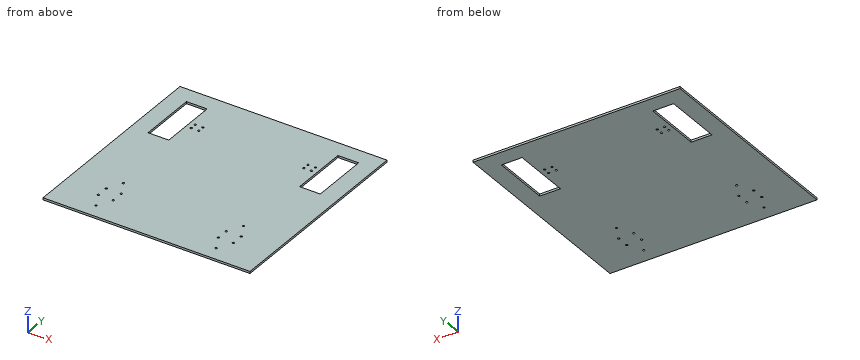
```python
from build123d import *

# Parameters (mm, degrees)
SKETCH1_W           = 500
SKETCH1_H           = 500
SKETCH1_R           = 2.5
SKETCH1_W_2         = 50
SKETCH1_H_2         = 140
BOSS_EXTRUDE1_DEPTH = 5
CUT_EXTRUDE1_START  = -5
SKETCH2_R           = 2.5
CUT_EXTRUDE1_DEPTH  = 5


with BuildPart() as part:
    # Sketch1 → Boss-Extrude1 (new body)
    with BuildSketch(Plane.XY):
        Rectangle(SKETCH1_W, SKETCH1_H)
        with Locations((127, 147.5)):
            Circle(SKETCH1_R, mode=Mode.SUBTRACT)
        with Locations((127, 132.5)):
            Circle(SKETCH1_R, mode=Mode.SUBTRACT)
        with Locations((145, 132.5)):
            Circle(SKETCH1_R, mode=Mode.SUBTRACT)
        with Locations((145, 147.5)):
            Circle(SKETCH1_R, mode=Mode.SUBTRACT)
        with Locations((-145, 147.5)):
            Circle(SKETCH1_R, mode=Mode.SUBTRACT)
        with Locations((-145, 132.5)):
            Circle(SKETCH1_R, mode=Mode.SUBTRACT)
        with Locations((-127, 132.5)):
            Circle(SKETCH1_R, mode=Mode.SUBTRACT)
        with Locations((-127, 147.5)):
            Circle(SKETCH1_R, mode=Mode.SUBTRACT)
        with Locations((183, 140)):
            Rectangle(SKETCH1_W_2, SKETCH1_H_2, mode=Mode.SUBTRACT)
        with Locations((-183, 140)):
            Rectangle(SKETCH1_W_2, SKETCH1_H_2, mode=Mode.SUBTRACT)
    extrude(amount=BOSS_EXTRUDE1_DEPTH)

    # Sketch2 → Cut-Extrude1 (cut)
    with BuildSketch(Plane.XY.offset(5).offset(CUT_EXTRUDE1_START)):
        with Locations((-145, 132.5)):
            Circle(SKETCH2_R)
        with Locations((-163.125, -150.6)):
            Circle(SKETCH2_R)
        with Locations((-126.875, -150.6)):
            Circle(SKETCH2_R)
        with Locations((-126.875, -179.4)):
            Circle(SKETCH2_R)
        with Locations((-163.125, -179.4)):
            Circle(SKETCH2_R)
        with Locations((-145, -115)):
            Circle(SKETCH2_R)
        with Locations((-145, -215)):
            Circle(SKETCH2_R)
        with Locations((145, -215)):
            Circle(SKETCH2_R)
        with Locations((145, -115)):
            Circle(SKETCH2_R)
        with Locations((163.125, -179.4)):
            Circle(SKETCH2_R)
        with Locations((126.875, -179.4)):
            Circle(SKETCH2_R)
        with Locations((126.875, -150.6)):
            Circle(SKETCH2_R)
        with Locations((163.125, -150.6)):
            Circle(SKETCH2_R)
    extrude(amount=CUT_EXTRUDE1_DEPTH, mode=Mode.SUBTRACT)


solid = part.part
```
For this review, take the finished solid that the model builds, in its own axes (mm). Round coordinates to 2 decimals unless told otherwise and drop trailing zeros. Write each loop counter-clockwise with the first axis right and the second up, starting at its lowest first coordinate (ties: lowest second). Pieces come first, ordered by that corner, then holes. Notation, with made-up numbers: (-13, 7.25) -> (10, 7.25) arc R34 ccw to (10, 41.25) -> close; hole circle Ø9 at (41.25, 35). An arc over 180 degrees is marked (long way). One line per question, with ' | ' between items. Start each with the question number.
(1) Insertion check: P1, Ø3, axis at x = -127, y = 132.5, coming from the -Z side. The pin has a flat end and moves straight along its axis. Give the tip position at first contact, or say it passes through.
(2) For line 1 along X through (y, z) = (173, 4.15); line 2 along X through (y, z) = (-150.6, 3.8) (3 decimals); line 3 along X through (y, z) = (-215, 2), list the stretches that pass through material, from the lowest coordinate up. Write a range as from..to.
(3) Add section B-B, the plane x = 180.5. Write out the cut boundary in (y, z), plus the area to 3 significant figures.
(4) Add section A-A, the plane y = 163.5. Write out the cut boundary in (x, z), plus the area to 3 significant figures.
Answer list:
1) P1: through
2) line 1: -250..-208, -158..158, 208..250 | line 2: -250..-165.625, -160.625..-129.375, -124.375..124.375, 129.375..160.625, 165.625..250 | line 3: -250..-147.5, -142.5..142.5, 147.5..250
3) outline: (-250, 0) -> (70, 0) -> (70, 5) -> (-250, 5) -> close; (210, 0) -> (250, 0) -> (250, 5) -> (210, 5) -> close | area: 1,800 mm²
4) outline: (-250, 0) -> (-208, 0) -> (-208, 5) -> (-250, 5) -> close; (-158, 0) -> (158, 0) -> (158, 5) -> (-158, 5) -> close; (208, 0) -> (250, 0) -> (250, 5) -> (208, 5) -> close | area: 2,000 mm²
